from build123d import *

# Parameters (mm, degrees)
SKETCH_1_R      = 27.5
SKETCH_1_R_2    = 10
EXTRUDE_1_DEPTH = 2
SKETCH_2_R      = 18
SKETCH_2_R_2    = 10
EXTRUDE_2_DEPTH = 24
SKETCH_3_R      = 27.5
SKETCH_3_R_2    = 10
EXTRUDE_3_DEPTH = 2
FILLET_1_R      = 0.5


with BuildPart() as part:
    # 草图1 → 凸台-拉伸1 (new body)
    with BuildSketch(Plane(origin=(0, 0, 0), x_dir=(1, 0, 0), z_dir=(0, 1, 0))):
        with Locations(Location((0, 0, 0), (0, 0, 270))):
            Circle(SKETCH_1_R)
        with Locations(Location((0, 0, 0), (0, 0, 270))):
            Circle(SKETCH_1_R_2, mode=Mode.SUBTRACT)
    extrude(amount=-EXTRUDE_1_DEPTH)

    # 草图2 → 凸台-拉伸2 (add)
    with BuildSketch(Plane.XZ.offset(2)):
        with Locations(Location((0, 0, 0), (0, 0, 90))):
            Circle(SKETCH_2_R)
        with Locations(Location((0, 0, 0), (0, 0, 90))):
            Circle(SKETCH_2_R_2, mode=Mode.SUBTRACT)
    extrude(amount=EXTRUDE_2_DEPTH)

    # 草图3 → 凸台-拉伸3 (add)
    with BuildSketch(Plane.XZ.offset(26)):
        with Locations(Location((0, 0, 0), (0, 0, 90))):
            Circle(SKETCH_3_R)
        with Locations(Location((0, 0, 0), (0, 0, 90))):
            Circle(SKETCH_3_R_2, mode=Mode.SUBTRACT)
    extrude(amount=EXTRUDE_3_DEPTH)

    # 圆角1
    fillet_1_edges = [part.edges().sort_by_distance(p)[0] for p in [
        (0, -28, -27.5),
        (0, -26, -27.5),
        (0, 0, -27.5),
        (0, -2, -27.5),
    ]]
    fillet(fillet_1_edges, radius=FILLET_1_R)


solid = part.part
Model file for the job. Use its own axes, mm. A direction names the side the tool comes from. Give positions to 0.01 mm unless a question says otherwise; leave off trailing zeros. Loops run counter-clockwise (first coordinate to the right, second up) from the corner with the lowest first, then second, coordinate; pieces in that order, holes last. Notation, with made-up numbers: (35, -7.5) -> (50, -7.5) arc R25 ccw to (50, 5.5) -> close; hole circle Ø6 at (-12, 54.5). An arc over 180 degrees is marked (long way). Use a Markdown table: item, result. Add a question column.
(1) Tool access for faces 1 (the cylindrical face through (-24.397, -0.993, 12.69)), 2 (the cylindrical face through (-5.407, -13.832, 17.169)): list every direction of +Z, -Z, +X, -X, +Y, -Y with a clear straight run to the whole face (end or side of a thin tool).
(2) Slice it at B-B on z = 0. List the corners of the cut face in (x, y).
(3) Drop flat-ended pins along their axis: pin 1 Ø10 at (y, z) = (-25, -4) entering from -X; pin 2 Ø12 at (x, z) = (0, 0) entering from -Y; pin 3 Ø10 at (x, y) = (-6.5, -15) entering from +Z; pin 4 Ø1.5 at (x, y) = (15.5, -14.5) entering from +Z. Give the stop position or say it passes through.
(4) Wall check: line 1 along X through (y, z) = (-0.65, 0); line 2 along Y through (x, z) = (-12.5, 16.5); line 3 along X through (y, z) = (-9.25, 0). Give the ranges that are in metal, low to high.
(5) Slice it at C-C on y = -17.75. List the corners of the cut face in (x, z), and give its area (3 significant figures).
(6) Slice it at A-A on x = 0. List the corners of the cut face in (y, z).
Filled sheet:
| question | item | result |
|---|---|---|
| 1 | face 1 | +Y, -Y |
| 1 | face 2 | none |
| 2 | outline | (-27.5, -27.5) arc R0.5 ccw to (-27, -28) -> (-10, -28) -> (-10, 0) -> (-27, 0) arc R0.5 ccw to (-27.5, -0.5) -> (-27.5, -1.5) arc R0.5 ccw to (-27, -2) -> (-18, -2) -> (-18, -26) -> (-27, -26) arc R0.5 ccw to (-27.5, -26.5) -> close; (10, -28) -> (27, -28) arc R0.5 ccw to (27.5, -27.5) -> (27.5, -26.5) arc R0.5 ccw to (27, -26) -> (18, -26) -> (18, -2) -> (27, -2) arc R0.5 ccw to (27.5, -1.5) -> (27.5, -0.5) arc R0.5 ccw to (27, 0) -> (10, 0) -> close |
| 3 | pin 1 | x = -27.5 |
| 3 | pin 2 | through |
| 3 | pin 3 | z = 17.94 |
| 3 | pin 4 | z = 10.32 |
| 4 | line 1 | -27.5 to -10, 10 to 27.5 |
| 4 | line 2 | -28 to -26, -2 to 0 |
| 4 | line 3 | -18 to -10, 10 to 18 |
| 5 | outline | circle Ø36 at (0, 0); hole circle Ø20 at (0, 0) |
| 5 | area | 704 mm2 |
| 6 | outline | (-28, -27) arc R0.5 ccw to (-27.5, -27.5) -> (-26.5, -27.5) arc R0.5 ccw to (-26, -27) -> (-26, -18) -> (-2, -18) -> (-2, -27) arc R0.5 ccw to (-1.5, -27.5) -> (-0.5, -27.5) arc R0.5 ccw to (0, -27) -> (0, -10) -> (-28, -10) -> close; (-28, 10) -> (0, 10) -> (0, 27) arc R0.5 ccw to (-0.5, 27.5) -> (-1.5, 27.5) arc R0.5 ccw to (-2, 27) -> (-2, 18) -> (-26, 18) -> (-26, 27) arc R0.5 ccw to (-26.5, 27.5) -> (-27.5, 27.5) arc R0.5 ccw to (-28, 27) -> close |
